Build history of the part. All positions in model axes, mm. Coordinates: 2 decimals unless noted, no trailing zeros. Write each loop counter-clockwise with the first axis right and the second up, starting at its lowest first coordinate (ties: lowest second). Pieces come first, ordered by that corner, then holes.
Autodesk Inventor part; units mm, degrees
ref_plane "YZ Plane" through (0, 0, 0) normal (1, 0, 0) x (0, 1, 0)
ref_plane "XZ Plane" through (0, 0, 0) normal (0, 1, 0) x (-1, 0, 0)
ref_plane "XY Plane" through (0, 0, 0) normal (0, 0, 1) x (1, 0, 0)
sketch "スケッチ1" plane through (0, 0, 0) normal (0, 1, 0) x (-1, 0, 0)
  circle A0 centre (0, 0) radius 5.7735
  line L0 (0, 0) -> (5, -2.8868)
  line L1 (5, -2.8868) -> (5, 0)
  line L2 (0, 0) -> (5, 0)
  line L3 (5, 2.8868) -> (5, 0)
  line L4 (5, 2.8868) -> (2.5, 4.3301)
  line L5 (0, 5.7735) -> (2.5, 4.3301)
  line L6 (0, 5.7735) -> (-2.5, 4.3301)
  line L7 (-5, 2.8868) -> (-2.5, 4.3301)
  line L8 (-5, 2.8868) -> (-5, 0)
  line L9 (-5, -2.8868) -> (-5, 0)
  line L10 (-5, -2.8868) -> (-2.5, -4.3301)
  line L11 (0, -5.7735) -> (-2.5, -4.3301)
  line L12 (0, -5.7735) -> (2.5, -4.3301)
  line L13 (5, -2.8868) -> (2.5, -4.3301)
  dimension "d1" = 5
  dimension "d2" = 30
  dimension "d5" = 360
extrude "押し出し1" add sketch "スケッチ1" along normal blind 10 contours L3 L2 L0 L13 L12 L11 L10 L9 L8 L7 L6 L5 L4 | L0 L2 L1
sketch "スケッチ2" plane through (0, 10, 0) normal (0, 1, 0) x (1, 0, 0)
  point P0 (0, 0)
  point P1 (0, 0)
hole "穴1" at (0, 10, 0) direction (0, -1, 0) diameter 4.2 end through all
properties part number "basespacer1" material "アルミニウム 6061"
(1) Slice it at B-B, the plane y = 5.25. List the corners of the cut face in (x, z), and give its area (3 significant figures).
(2) Slice it at A-A, the plane z = 0. List the corners of the cut face in (x, y).
(3) Flat gauge pins, fed straight in: P1, Ø3, axis at x = -1, y = 3, coming from the -Z side; P2, Ø1.5, axis at x = 3.5, y = 3.5, coming from the -Z side. Where does each tip first touch, or does it go through?
(4) Slice it at D-D, the plane z = 3.5. List the corners of the cut face in (x, y), and give its area (3 significant figures).
(5) Slice it at C-C, the plane z = 1.75. List the corners of the cut face in (x, y).
(6) Probe L1, parallel to X at y = 7.5, z = 0; L2, parallel to Z at x = 0.75, y = 9; L3, parallel to Z at x = -1.5, y = 0.5. List the from-to ranges inside material, lowest first.
(7) Two-plate mould, pull along X, no slides. Class faces 1 (the cylindrical face through (-0.631, 4.93, 2.003)), 2 (the flat face through (-5, 5, 0)), 3 (the flat face through (5, 5, 0)): pulls with the +X half, pulls with the -X half, needs draft (parallel to the pull), parting line crosses it, or undercut.
Results:
1. outline: (-5, -2.89) - (-2.5, -4.33) - (0, -5.77) - (2.5, -4.33) - (5, -2.89) - (5, 2.89) - (2.5, 4.33) - (0, 5.77) - (-2.5, 4.33) - (-5, 2.89) - close; hole circle Ø4.2 at (0, 0)
1. area: 72.7 mm2
2. outline: (-5, 0) - (-2.1, 0) - (-2.1, 10) - (-5, 10) - close; (2.1, 0) - (5, 0) - (5, 10) - (2.1, 10) - close
3. P1: stops at z = -5.77
3. P2: stops at z = -4.19
4. outline: (-3.94, 0) - (3.94, 0) - (3.94, 10) - (-3.94, 10) - close
4. area: 78.8 mm2
5. outline: (-5, 0) - (-1.16, 0) - (-1.16, 10) - (-5, 10) - close; (1.16, 0) - (5, 0) - (5, 10) - (1.16, 10) - close
6. L1: x = -5 to -2.1, 2.1 to 5
6. L2: z = -5.34 to -1.96, 1.96 to 5.34
6. L3: z = -4.91 to -1.47, 1.47 to 4.91
7. face 1: undercut
7. face 2: pulls with the -X half
7. face 3: pulls with the +X half
